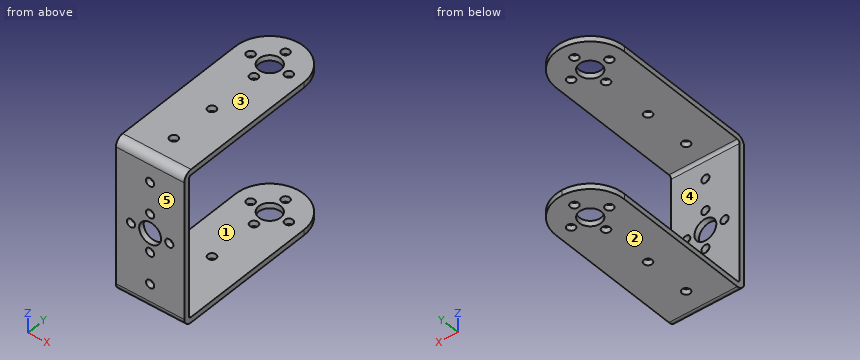
```python
from build123d import *

# Parameters (mm, degrees)
BASE_FLANGE1_DEPTH           = 2
EDGE_FLANGE1_DEPTH           = 25
EDGE_FLANGE2_STRIP_W         = 10
EDGE_FLANGE2_STRIP_H         = 2
EDGE_FLANGE2_STRIP_CUT_DEPTH = 25
EDGE_FLANGE2_DEPTH           = 25
CUT_EXTRUDE1_START           = -2
CUT_EXTRUDE1_DEPTH           = 2
SKETCH19_R                   = 4
CUT_EXTRUDE2_DEPTH           = 85.843974447
M3X0_5_TAPPED_HOLE1_D        = 3
SKETCH22_R                   = 4
CUT_EXTRUDE3_DEPTH           = 86.583292762
M3X0_5_TAPPED_HOLE2_D        = 3


# Sheet-metal steps are written as plain solids
with BuildPart() as part:
    # Sketch8 → Base-Flange1 (new body)
    with BuildSketch(Plane.XY):
        with BuildLine():
            Line((-12.5, 0), (12.5, 0))
            Line((12.5, 0), (12.5, 50))
            ThreePointArc((12.5, 50), (0, 62.5), (-12.5, 50))
            Line((-12.5, 50), (-12.5, 0))
        make_face()
    extrude(amount=-BASE_FLANGE1_DEPTH)

    # Edge-Flange1 section (across the edge) → Edge-Flange1 (add)
    with BuildSketch(Plane(origin=(12.5, -1, -2), x_dir=(0, 1, 0), z_dir=(-1, 0, 0))):
        with BuildLine():
            Line((-2, 1), (-2, 52))
            Line((-2, 52), (0, 52))
            Line((0, 52), (0, 1))
            ThreePointArc((0, 1), (0.292893219, 0.292893219), (1, 0))
            Line((1, 0), (1, -2))
            ThreePointArc((1, -2), (-1.121320344, -1.121320344), (-2, 1))
        make_face()
    extrude(amount=EDGE_FLANGE1_DEPTH)

    # Edge-Flange2 strip (across the edge) → Edge-Flange2 strip cut (cut)
    with BuildSketch(Plane(origin=(12.5, -1, -54), x_dir=(0, 0, 1), z_dir=(-1, 0, 0))):
        with Locations((-4, -1)):
            Rectangle(EDGE_FLANGE2_STRIP_W, EDGE_FLANGE2_STRIP_H)
    extrude(amount=EDGE_FLANGE2_STRIP_CUT_DEPTH, mode=Mode.SUBTRACT)

    # Edge-Flange2 section (across the edge) → Edge-Flange2 (add)
    with BuildSketch(Plane(origin=(12.5, -1, -54), x_dir=(0, 0, 1), z_dir=(-1, 0, 0))):
        with BuildLine():
            Line((-2, 1), (-2, 63.5))
            Line((-2, 63.5), (0, 63.5))
            Line((0, 63.5), (0, 1))
            ThreePointArc((0, 1), (0.292893219, 0.292893219), (1, 0))
            Line((1, 0), (1, -2))
            ThreePointArc((1, -2), (-1.121320344, -1.121320344), (-2, 1))
        make_face()
    extrude(amount=EDGE_FLANGE2_DEPTH)

    # Sketch18 → Cut-Extrude1 (cut)
    with BuildSketch(Plane(origin=(0, 0, -56), x_dir=(-1, 0, 0), z_dir=(0, 0, -1)).offset(CUT_EXTRUDE1_START)):
        with BuildLine():
            ThreePointArc((0, 62.5), (8.838834765, 58.838834765), (12.5, 50))
            Line((12.5, 50), (12.5, 62.5))
            Line((12.5, 62.5), (0, 62.5))
        make_face()
        with BuildLine():
            ThreePointArc((-12.5, 50), (-8.838834765, 58.838834765), (0, 62.5))
            Line((0, 62.5), (-12.5, 62.5))
            Line((-12.5, 62.5), (-12.5, 50))
        make_face()
    extrude(amount=CUT_EXTRUDE1_DEPTH, mode=Mode.SUBTRACT)

    # Sketch19 → Cut-Extrude2 (cut, through all)
    with BuildSketch(Plane.XY):
        with Locations((0, 50)):
            Circle(SKETCH19_R)
    extrude(amount=-CUT_EXTRUDE2_DEPTH, mode=Mode.SUBTRACT)

    # M3x0.5 Tapped Hole1 (through all)
    with Locations(Plane.XY):
        with Locations((0, 57), (-7, 50), (0, 43), (7, 50), (0, 24.4), (0, 7.53)):
            Hole(M3X0_5_TAPPED_HOLE1_D / 2)

    # Sketch22 → Cut-Extrude3 (cut, through all)
    with BuildSketch(Plane(origin=(0, -1, 0), x_dir=(1, 0, 0), z_dir=(0, 1, 0))):
        with Locations(Location((0, 28, 0), (0, 0, 270))):
            Circle(SKETCH22_R)
    extrude(amount=-CUT_EXTRUDE3_DEPTH, mode=Mode.SUBTRACT)

    # M3x0.5 Tapped Hole2 (through all)
    with Locations(Plane(origin=(0, -1, 0), x_dir=(1, 0, 0), z_dir=(0, 1, 0))):
        with Locations((7, 28), (-7, 28), (0, 35), (0, 21), (0, 9.4), (0, 46.6)):
            Hole(M3X0_5_TAPPED_HOLE2_D / 2)


solid = part.part
```
Source: CAD feature listing. Evaluate the final solid. Frame: model axes, mm. Face numbers are marked on the shaded views. A direction names the side the tool comes from. Coordinates: 2 decimals unless noted, no trailing zeros. Loops run counter-clockwise (first coordinate to the right, second up) from the corner with the lowest first, then second, coordinate; pieces in that order, holes last. Notation, with made-up numbers: (32, -10.5) -> (73, -10.5) arc R31 cw to (73, 24.5) -> close; hole circle Ø2 at (87, -34.75). An arc over 180 degrees is marked (long way). One line per item, written item: value. Start each with the question number.
Q1. Line query: line 1 along Z through (x, y) = (10, 13.5); line 2 along Y through (x, z) = (0, -55.05); line 3 along Y through (x, z) = (-5.75, -6). Output: solid intervals per line, ascending.
Q2. Section query D-D, the plane z = -28. Return the cut outline in (x, y), and give its area (3 significant figures).
Q3. Mould query, pull axis Z, two halves, no side actions, for the marked faces 1, 2 and 3. Classes: pulls with the +Z half, pulls with the -Z half, needs draft (parallel to the pull), parting line crosses it, or undercut.
Q4. Section query B-B, the plane y = 14. Return the cut outline in (x, z), and give its area (3 significant figures).
Q5. Section query A-A, the plane z = -46.6. Return the cut outline in (x, y), and give its area (3 significant figures).
Q6. Contact query for flat-ended pins moving along their axis: P1, Ø2.5, axis at x = -7, z = -28, coming from the +Y side; P2, Ø1, axis at x = -2.5, z = -49.5, coming from the +Y side. Output: stop coordinate, or through.
Q7. Section query C-C, the plane x = 7.25. Return the cut outline in (y, z), and give its area (3 significant figures).
Q8. Set-up query: the marked faces 4 and 5. Return all of +Z, -Z, +X, -X, +Y, -Y with unobstructed straight access to the full face (end or side cutting, diameter ignored); none if empty.
Results:
1. line 1: -56 to -54, -2 to 0
1. line 2: -2.19 to 6.03, 9.03 to 22.9, 25.9 to 41.5, 44.5 to 46, 54 to 55.5, 58.5 to 62.5
1. line 3: -3 to -1
2. outline: (-12.5, -3) -> (-8.5, -3) -> (-8.5, -1) -> (-12.5, -1) -> close; (-5.5, -3) -> (-4, -3) -> (-4, -1) -> (-5.5, -1) -> close; (4, -3) -> (5.5, -3) -> (5.5, -1) -> (4, -1) -> close; (8.5, -3) -> (12.5, -3) -> (12.5, -1) -> (8.5, -1) -> close
2. area: 22.0 mm^2
3. face 1: undercut
3. face 2: pulls with the -Z half
3. face 3: pulls with the +Z half
4. outline: (-12.5, -56) -> (12.5, -56) -> (12.5, -54) -> (-12.5, -54) -> close; (-12.5, -2) -> (12.5, -2) -> (12.5, 0) -> (-12.5, 0) -> close
4. area: 100 mm^2
5. outline: (-12.5, -3) -> (-1.5, -3) -> (-1.5, -1) -> (-12.5, -1) -> close; (1.5, -3) -> (12.5, -3) -> (12.5, -1) -> (1.5, -1) -> close
5. area: 44.0 mm^2
6. P1: through
6. P2: y = -1
7. outline: (-3, -53) arc R3 ccw to (0, -56) -> (48.52, -56) -> (48.52, -54) -> (0, -54) arc R1 cw to (-1, -53) -> (-1, -29.48) -> (-3, -29.48) -> close; (-3, -26.52) -> (-1, -26.52) -> (-1, -3) arc R1 cw to (0, -2) -> (48.52, -2) -> (48.52, 0) -> (0, 0) arc R3 ccw to (-3, -3) -> close; (51.48, -56) -> (60.18, -56) -> (60.18, -54) -> (51.48, -54) -> close; (51.48, -2) -> (60.18, -2) -> (60.18, 0) -> (51.48, 0) -> close
7. area: 336 mm^2
8. face 4: +X, -X, +Y
8. face 5: +Z, -Z, +X, -X, -Y
